from build123d import *

# Parameters (mm, degrees)
ESBO_O1_R                = 5.25
RESSALTO_EXTRUS_O1_DEPTH = 3
FILETE1_R                = 15
ESBO_O2_W                = 3
ESBO_O2_H                = 35
CORTE_EXTRUS_O1_DEPTH    = 3


with BuildPart() as part:
    # Esboço1 → Ressalto-extrusão1 (new body)
    with BuildSketch(Plane.XY):
        with BuildLine():
            Line((-23.5, 0), (-16.5, 0))
            Line((-16.5, 0), (-16.5, 3))
            Line((-16.5, 3), (16.5, 3))
            Line((16.5, 3), (16.5, 0))
            Line((16.5, 0), (23.5, 0))
            Line((23.5, 0), (23.5, 12))
            Line((23.5, 12), (4.5, 92))
            Line((4.5, 92), (4.5, 104))
            ThreePointArc((4.5, 104), (6.708203932, 106.645898034), (7.5, 110))
            Line((7.5, 110), (7.5, 155))
            ThreePointArc((7.5, 155), (0, 162.5), (-7.5, 155))
            Line((-7.5, 155), (-7.5, 110))
            ThreePointArc((-7.5, 110), (-6.708203932, 106.645898034), (-4.5, 104))
            Line((-4.5, 104), (-4.5, 92))
            Line((-4.5, 92), (-23.5, 12))
            Line((-23.5, 12), (-23.5, 0))
        make_face()
        with Locations((0, 110)):
            Circle(ESBO_O1_R, mode=Mode.SUBTRACT)
        with Locations((0, 125)):
            Circle(ESBO_O1_R, mode=Mode.SUBTRACT)
        with Locations((0, 140)):
            Circle(ESBO_O1_R, mode=Mode.SUBTRACT)
        with Locations((0, 155)):
            Circle(ESBO_O1_R, mode=Mode.SUBTRACT)
    extrude(amount=RESSALTO_EXTRUS_O1_DEPTH)

    # Filete1
    filete1_edges = [part.edges().sort_by_distance(p)[0] for p in [
        (-23.5, 12, 1.5),
        (-4.5, 92, 1.5),
        (-4.5, 104, 1.5),
        (4.5, 104, 1.5),
        (4.5, 92, 1.5),
        (23.5, 12, 1.5),
    ]]
    fillet(filete1_edges, radius=FILETE1_R)

    # Esboço2 → Corte-extrusão1 (cut)
    with BuildSketch(Plane.XY.offset(3)):
        with Locations((0, 20.5)):
            Rectangle(ESBO_O2_W, ESBO_O2_H)
    extrude(amount=-CORTE_EXTRUS_O1_DEPTH, mode=Mode.SUBTRACT)


solid = part.part
CAD build for the part. Positions are in the model's coordinates, mm. A direction names the side the tool comes from. Coordinates: 2 decimals unless noted, no trailing zeros. Order: outer loops, then holes, each group sorted by start corner. A loop starts at its lowest first (then second) coordinate and runs counter-clockwise, first axis right, second up.
Item 1: Two-plate mould, pull along X, no slides. Class faces 4 (the face through (-20, 0, 1)), 5 (the face through (-1.138, 134.875, 1.479)), 6 (the face through (7.24, 108.04, 1.48)): +X half, -X half, draft (parallel to the pull), parting line (faces both ways), or undercut.
Check sheet entries:
face 4: draft
face 5: undercut
face 6: +X half
Item 2: Band-saw the part on D-D on x = 15. List the corners of the cut face in (y, z), plus the area to 3 significant figures.
Check sheet entries:
outline: (3, 0) - (47.79, 0) - (47.79, 3) - (3, 3) - close
area: 134 mm2
Item 3: Band-saw the part on A-A on x = 0. List the corners of the cut face in (y, z), plus the area to 4 significant figures.
Check sheet entries:
outline: (38, 0) - (104.75, 0) - (104.75, 3) - (38, 3) - close; (115.25, 0) - (119.75, 0) - (119.75, 3) - (115.25, 3) - close; (130.25, 0) - (134.75, 0) - (134.75, 3) - (130.25, 3) - close; (145.25, 0) - (149.75, 0) - (149.75, 3) - (145.25, 3) - close; (160.25, 0) - (162.5, 0) - (162.5, 3) - (160.25, 3) - close
area: 247.5 mm2
Item 4: Band-saw the part on B-B on y = 125. List the corners of the cut face in (x, z), plus the area to 3 significant figures.
Check sheet entries:
outline: (-7.5, 0) - (-5.25, 0) - (-5.25, 3) - (-7.5, 3) - close; (5.25, 0) - (7.5, 0) - (7.5, 3) - (5.25, 3) - close
area: 13.5 mm2
Item 5: Band-saw the part on C-C on z = 1.9. Give the number of separate pieces and of enclosed holes in the cut face, plus the area to 3 significant figures.
Check sheet entries:
separate pieces: 1
enclosed holes: 4
area: 3,210 mm2
Item 6: 3-axis set-ups, long thin cutter, end or side, ignore diameter. For faces 1 (the face through (-4.995, 102.595, 1.521)), 2 (the face through (0, 38, 2)), 3 (the face through (0, 64, 0)): which of +Z, -Z, +X, -X, +Y, -Y reach the whole face in a straight line?
Check sheet entries:
face 1: +Z, -Z, -X
face 2: +Z, -Z, -Y
face 3: -Z, +X, -X, +Y, -Y
Item 7: Pin check, flat tips, straight feed: pin 1 Ø1.5 at (x, z) = (-12.5, 1) entering from -Y; pin 2 Ø0.9 at (y, z) = (95.5, 1) entering from +X; pin 3 Ø1 at (y, z) = (129, 1.5) entering from +X. Stop position of each tip, or through.
Check sheet entries:
pin 1: stops at y = 3
pin 2: stops at x = 4.5
pin 3: stops at x = 7.5
Item 8: Drill centre lines: L1, parallel to Y at x = 0, z = 0.8; L2, parallel to X at y = 10.5, z = 2.5; L3, parallel to X at y = 155.5, z = 0.95. Where is each one in solid material? Low to high.
Check sheet entries:
L1: y = 38 to 104.75, 115.25 to 119.75, 130.25 to 134.75, 145.25 to 149.75, 160.25 to 162.5
L2: x = -23.5 to -1.5, 1.5 to 23.5
L3: x = -7.48 to -5.23, 5.23 to 7.48
